```python
from build123d import *

# Parameters (mm, degrees)
F0_W      = 84.451213479
F0_H      = 112.9794791341
F1_DEPTH  = 25.4
F2_W      = 50.8853495121
F2_H      = 82.8240290284
F3_DEPTH  = 25.4
F4_R      = 6.2891485283
F5_DEPTH  = 25.4
F6_R      = 5.5560325186
F7_DEPTH  = 25.4
F8_W      = 17.1270668507
F8_H      = 18.73687841
F9_DEPTH  = 12.7
F10_W     = 16.4387971163
F10_H     = 65.7989624888
F11_DEPTH = 12.7


with BuildPart() as f1:
    # F0 (on Top) → F1 (new body)
    with BuildSketch(Plane.XY):
        with Locations((3.9865151048, 3.3602751791)):
            Rectangle(F0_W, F0_H)
    extrude(amount=F1_DEPTH)

    # F2 (on face) → F3 (cut)
    with BuildSketch(Plane.XY.offset(25.4)):
        with Locations((4.330649972, 2.2555477917)):
            Rectangle(F2_W, F2_H)
    extrude(amount=-F3_DEPTH, mode=Mode.SUBTRACT)

    # F4 (on face) → F5 (cut)
    with BuildSketch(Plane(origin=(0, 59.8500147462, 0), x_dir=(-1, 0, 0), z_dir=(0, 1, 0))):
        with Locations((-5.7790102437, 17.3808317631)):
            Circle(F4_R)
    extrude(amount=-F5_DEPTH, mode=Mode.SUBTRACT)

    # F6 (on face) → F7 (cut)
    with BuildSketch(Plane.XZ.offset(53.1294643879)):
        with Locations((3.0174842104, 10.6666553766)):
            Circle(F6_R)
    extrude(amount=-F7_DEPTH, mode=Mode.SUBTRACT)

    # F8 (on face) → F9 (cut)
    with BuildSketch(Plane(origin=(0, 0, 0), x_dir=(1, 0, 0), z_dir=(0, 0, -1))):
        with Locations((-29.6755582094, -1.4471039176)):
            Rectangle(F8_W, F8_H)
    extrude(amount=-F9_DEPTH, mode=Mode.SUBTRACT)

    # F10 (on face) → F11 (cut)
    with BuildSketch(Plane(origin=(0, 0, 0), x_dir=(1, 0, 0), z_dir=(0, 0, -1))):
        with Locations((37.9927232862, -5.4467311129)):
            Rectangle(F10_W, F10_H)
    extrude(amount=-F11_DEPTH, mode=Mode.SUBTRACT)


solid = f1.part
```
The model under review builds one solid part; all positions refer to its coordinate system, in mm. A direction names the side the tool comes from. Round coordinates to 2 decimals unless told otherwise and drop trailing zeros. Loops run counter-clockwise (first coordinate to the right, second up) from the corner with the lowest first, then second, coordinate; pieces in that order, holes last. Notation, with made-up numbers: (34, 5.5) -> (41, 5.5) arc R5 cw to (41, 13.5) -> close; hole circle Ø7 at (-31, 0). An arc over 180 degrees is marked (long way). Answer in a Markdown table with one row per item.
1) Consider section C-C, the plane z = 8.25. Write out the cut boundary in (x, y).
Taken from the geometry:
| item | result |
|---|---|
| outline | (-38.24, -53.13) -> (-1.99, -53.13) -> (-1.99, -39.16) -> (-21.11, -39.16) -> (-21.11, -7.92) -> (-38.24, -7.92) -> close; (-38.24, 10.82) -> (-21.11, 10.82) -> (-21.11, 43.67) -> (29.77, 43.67) -> (29.77, 38.35) -> (46.21, 38.35) -> (46.21, 59.85) -> (-38.24, 59.85) -> close; (8.02, -53.13) -> (46.21, -53.13) -> (46.21, -27.45) -> (29.77, -27.45) -> (29.77, -39.16) -> (8.02, -39.16) -> close |
2) Consider section A-A, the plane y = 26. Write out the cut boundary in (x, z).
Taken from the geometry:
| item | result |
|---|---|
| outline | (-38.24, 0) -> (-21.11, 0) -> (-21.11, 25.4) -> (-38.24, 25.4) -> close; (29.77, 12.7) -> (46.21, 12.7) -> (46.21, 25.4) -> (29.77, 25.4) -> close |
3) For pin 1 Ø8 at (x, y) = (39.5, 6.5) entering from -Z, flat-tipped, find the tip position at first contact; note if it passes through.
Taken from the geometry:
| item | result |
|---|---|
| pin 1 | stops at z = 12.7 |
4) Draft analysis for pull direction Y (two halves, no side actions). For faces 4 (the flat face through (3, -53.129, 18)), 5 (the flat face through (38, 5, 12.7)), 6 (the cylindrical face through (2.294, -46.241, 16.175)), state which applies: pulls with the +Y half, pulls with the -Y half, needs draft (parallel to the pull), parting line crosses it, or undercut.
Taken from the geometry:
| item | result |
|---|---|
| face 4 | pulls with the -Y half |
| face 5 | undercut |
| face 6 | needs draft |
5) Consider section D-D, the plane x = -28.5. Write out the cut boundary in (y, z), plus the area to 3 significant figures.
Taken from the geometry:
| item | result |
|---|---|
| outline | (-53.13, 0) -> (-7.92, 0) -> (-7.92, 12.7) -> (10.82, 12.7) -> (10.82, 0) -> (59.85, 0) -> (59.85, 25.4) -> (-53.13, 25.4) -> close |
| area | 2,630 mm² |
6) Consider section B-B, the plane x = -19.5. Write out the cut boundary in (y, z).
Taken from the geometry:
| item | result |
|---|---|
| outline | (-53.13, 0) -> (-39.16, 0) -> (-39.16, 25.4) -> (-53.13, 25.4) -> close; (43.67, 0) -> (59.85, 0) -> (59.85, 25.4) -> (43.67, 25.4) -> close |
7) Wall thickness on line 1 along X through (y, z) = (-37, 9.75); line 2 along Y through (x, z) = (38, 6); line 3 along Y through (x, z) = (-13, 7.75): over which ranges is each line inside the solid? List them lowest first.
Taken from the geometry:
| item | result |
|---|---|
| line 1 | x = -38.24 to -21.11, 29.77 to 46.21 |
| line 2 | y = -53.13 to -27.45, 38.35 to 59.85 |
| line 3 | y = -53.13 to -39.16, 43.67 to 59.85 |
8) Tool access review of faces 1 (the flat face through (38, -27.453, 6)), 2 (the flat face through (-30, 10.816, 6)), 3 (the flat face through (10, -39.156, 13)): name each direction out of +Z, -Z, +X, -X, +Y, -Y from which nothing blocks a thin tool from reaching the whole face with its end or side.
Taken from the geometry:
| item | result |
|---|---|
| face 1 | -Z, +X |
| face 2 | -Z, +X, -X |
| face 3 | +Z, -Z |
